Could you check a few things on this drawing? It's one solid part, dimensions in mm from its lowest x, y, z. A direction names the side the tool comes from. Give positions to 0.01 mm unless a question says otherwise; leave off trailing zeros. Loops run counter-clockwise (first coordinate to the right, second up) from the corner with the lowest first, then second, coordinate; pieces in that order, holes last.
Q1. Suppose I cut it at D-D (y = 6). List the corners of the cut face in (x, z) for me.
Q2. I'm going to push flat-ended pins straight in: P1, Ø0.9, axis at y = 16, z = 6.5, coming from the +X side; P2, Ø6, axis at x = 31, y = 15, coming from the +Z side; P3, Ø1.5, axis at y = 6, z = 6, coming from the -X side. Where does each tip first touch, or does it pass through?
Q3. Suppose I cut it at C-C (z = 2.5). List the corners of the cut face in (x, y) for me.
Q4. Suppose I cut it at A-A (z = 6.75). List the corners of the cut face in (x, y) for me, and give its area (3 significant figures).
Q5. Thinking about a two-plate mould opening in Y: for the marked faces 1, 2 and 3, which applies, pulls with the +Y half, pulls with the -Y half, needs draft (parallel to the pull), parting line crosses it, or undercut?
Q6. For the marked faces 4, 5 and 6, which set-ups out of +Z, -Z, +X, -X, +Y, -Y let a thin tool reach every point of the face, with its end or its side?
Q7. I need wall thicknesses on probe 1 along X at (y, z) = (19, 0.8); probe 2 along Y at (x, z) = (5, 0.8); probe 3 along Y at (x, z) = (44, 0.95). Which ranges of each line are inside material? Lowest first, please.
Q8. Suppose I cut it at B-B (x = 5). List the corners of the cut face in (y, z) for me.
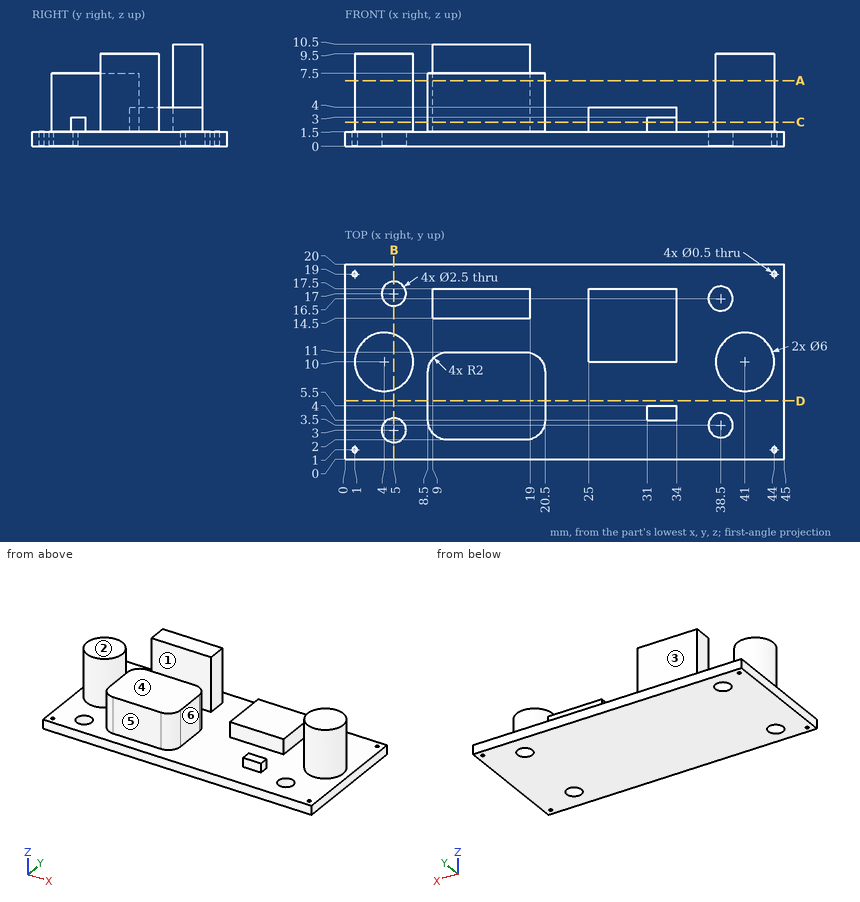
Solutions:
1. outline: (0, 0) - (45, 0) - (45, 1.5) - (20.5, 1.5) - (20.5, 7.5) - (8.5, 7.5) - (8.5, 1.5) - (0, 1.5) - close
2. P1: stops at x = 19
2. P2: stops at z = 4
2. P3: stops at x = 8.5
3. outline: circle Ø6 at (4, 10); (8.5, 4) arc R2 ccw to (10.5, 2) - (18.5, 2) arc R2 ccw to (20.5, 4) - (20.5, 9) arc R2 ccw to (18.5, 11) - (10.5, 11) arc R2 ccw to (8.5, 9) - close; (9, 14.5) - (19, 14.5) - (19, 17.5) - (9, 17.5) - close; (25, 10) - (34, 10) - (34, 17.5) - (25, 17.5) - close; (31, 4) - (34, 4) - (34, 5.5) - (31, 5.5) - close; circle Ø6 at (41, 10)
4. outline: circle Ø6 at (4, 10); (8.5, 4) arc R2 ccw to (10.5, 2) - (18.5, 2) arc R2 ccw to (20.5, 4) - (20.5, 9) arc R2 ccw to (18.5, 11) - (10.5, 11) arc R2 ccw to (8.5, 9) - close; (9, 14.5) - (19, 14.5) - (19, 17.5) - (9, 17.5) - close; circle Ø6 at (41, 10)
4. area: 191 mm2
5. face 1: undercut
5. face 2: needs draft
5. face 3: pulls with the +Y half
6. face 4: +Z, -Y
6. face 5: +Z, +X, -X, -Y
6. face 6: +Z, +Y, -Y
7. probe 1: x = 0 to 0.75, 1.25 to 43.75, 44.25 to 45
7. probe 2: y = 0 to 1.75, 4.25 to 15.75, 18.25 to 20
7. probe 3: y = 0 to 0.75, 1.25 to 18.75, 19.25 to 20
8. outline: (0, 0) - (1.75, 0) - (1.75, 1.5) - (0, 1.5) - close; (4.25, 0) - (15.75, 0) - (15.75, 1.5) - (12.83, 1.5) - (12.83, 9.5) - (7.17, 9.5) - (7.17, 1.5) - (4.25, 1.5) - close; (18.25, 0) - (20, 0) - (20, 1.5) - (18.25, 1.5) - close
